CAD build for the part. Positions are in the model's coordinates, mm. A direction names the side the tool comes from. Give positions to 0.01 mm unless a question says otherwise; leave off trailing zeros. Loops run counter-clockwise (first coordinate to the right, second up) from the corner with the lowest first, then second, coordinate; pieces in that order, holes last. Notation, with made-up numbers: M 74.25,-29 L 83.25,-29 A16 cw 83.25,-16 Z; hole C 80,10.25 d3. An arc over 180 degrees is marked long. Answer as CSV lines item,"result".
```python
from build123d import *

# Parameters (mm, degrees)
F0_W     = 285.75
F0_H     = 12.7
F0_R     = 31.829375
F1_DEPTH = 25


# Not quite as in the source:
# - ends of sketch curves that miss each other by under 0.0002 mm in the source are joined


with BuildPart() as f1:
    # F0 (on Right) → F1 (new body)
    with BuildSketch(Plane.YZ):
        with Locations((-174.078946, 333.521804)):
            Rectangle(F0_W, F0_H)
        with BuildLine():
            Line((-316.953946, 339.871804), (-31.203946, 339.871804))
            Line((-31.203946, 339.871804), (-21.297946, 339.871804))
            Line((-21.297946, 339.871804), (-21.297946, 431.783595))
            ThreePointArc((-21.297946, 431.783595), (-36.138421464, 465.080578536), (-69.4354049904, 479.9210541806))
            Line((-69.4354049904, 479.9210541806), (-326.859946, 479.921054))
            Line((-326.859946, 479.921054), (-326.859946, 339.871804))
            Line((-326.859946, 339.871804), (-316.953946, 339.871804))
        make_face()
        with Locations((-72.140054, 429.078946)):
            Circle(F0_R, mode=Mode.SUBTRACT)
    extrude(amount=F1_DEPTH)


solid = f1.part
```
Q1. Cut at A-A (z = 455). Write the cut outline in (x, y).
Solution:
outline,"M 0,-326.86 L 25,-326.86 L 25,-90.61 L 0,-90.61 Z; M 0,-53.67 L 25,-53.67 L 25,-28.32 L 0,-28.32 Z"
Q2. Cut at C-C (y = -79). Write the cut outline in (x, z).
Solution:
outline,"M 0,327.17 L 25,327.17 L 25,398 L 0,398 Z; M 0,460.16 L 25,460.16 L 25,479.92 L 0,479.92 Z"
Q3. Mould opens along Z. For faces 1 (the flat face through (12, -322, 339.872)), 2 (the flat face through (12, -316.954, 333)), 3 (the cylindrical face through (12.3, -55, 455.9)) say: released by +Z, released by -Z, zero draft, split by the parting line, or undercut.
Solution:
face 1,"released by -Z"
face 2,"zero draft"
face 3,"undercut"
Q4. Pin check, flat tips, straight feed: P1, Ø6.5, axis at x = 9.5, z = 333.5, coming from the +Y side; P2, Ø3, axis at x = 7.5, y = -324.5, coming from the -Z side; P3, Ø10, axis at x = 9.5, z = 330.5, coming from the -Y side; P4, Ø1, axis at y = -180, z = 428, coming from the -X side. Stop position of each tip, or through.
Solution:
P1,"stops at y = -31.2"
P2,"stops at z = 339.87"
P3,"stops at y = -316.95"
P4,"stops at x = 0"
Q5. Wall check: line 1 (Z direction, x = 1.75, y = -81.5); line 2 (Y direction, x = 12, z = 414); line 3 (Y direction, x = 7, z = 421). Give the ranges that are in metal, low to high. Write a range as [from, to].
Solution:
line 1,"z = [327.17, 398.66], [459.5, 479.92]"
line 2,"y = [-326.86, -100.17], [-44.11, -21.3]"
line 3,"y = [-326.86, -102.93], [-41.35, -21.3]"
Q6. Cut at B-B (x = 10.75). Write the cut outline in (y, z).
Solution:
outline,"M -326.86,339.87 L -316.95,339.87 L -316.95,327.17 L -31.2,327.17 L -31.2,339.87 L -21.3,339.87 L -21.3,431.78 A50.91 ccw -69.44,479.92 L -326.86,479.92 Z; hole C -72.14,429.08 d63.66"
Q7. Which spindle directions (+Z, -Z, +X, -X, +Y, -Y) get a long thin tool onto all of the face, cutting with end or side? Do faces 4 (the cylindrical face through (12.32, -35.77, 464.71)), 5 (the flat face through (12, -31.204, 333)). Say none if no direction does.
Solution:
face 4,"+Z, +X, -X, +Y"
face 5,"-Z, +X, -X, +Y"
